Here's the drawing with two shaded views (mm, measured from the low corner). I have some questions. Round coordinates to 2 decimals unless told otherwise and drop trailing zeros. Order: outer loops, then holes, each group sorted by start corner. A loop starts at its lowest first (then second) coordinate and runs counter-clockwise, first axis right, second up. Notation, with made-up numbers: (68.5, 39) -> (127.5, 39) arc R27 cw to (127.5, 69) -> close; hole circle Ø7 at (-7, 69). An arc over 180 degrees is marked (long way). Use a Markdown table: item, result. Add a question column.
Q1. If we section it at A-A on y = 83: List the corners of the cut face in (x, z) for me (3 decimals), plus the area to 3 significant figures.
Q2. I'm going to push a flat-ended pin straight in: pin 1 Ø4 at (x, y) = (17, 192) entering from -Z. Where does the tip first touch, or does it pass through?
Q3. I need wall thicknesses on line 1 along Z through (x, y) = (15, 193.5) (3 decimals); line 2 along X through (y, z) = (268, 28.5). Which ranges of each line are inside material? Lowest first, please. Write a range as [from, to].
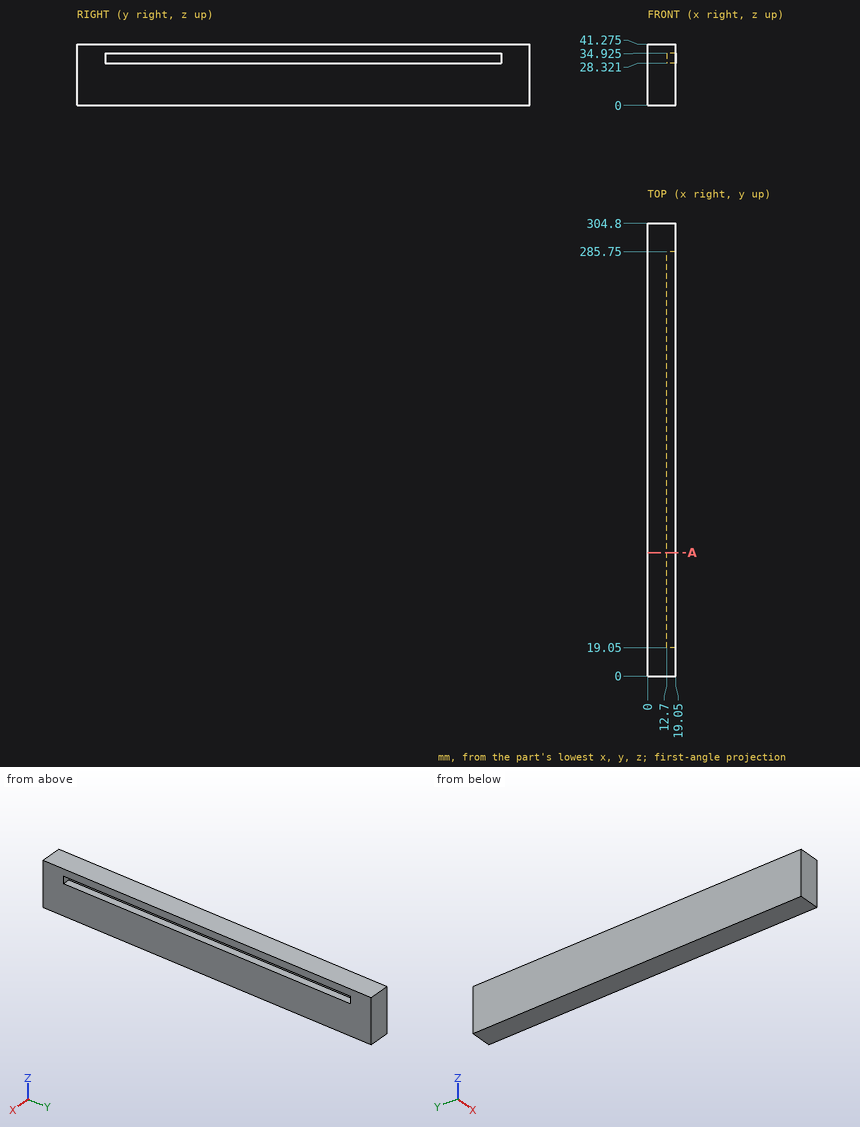
Answer below:
| question | item | result |
|---|---|---|
| 1 | outline | (0, 0) -> (19.05, 0) -> (19.05, 28.321) -> (12.7, 28.321) -> (12.7, 34.925) -> (19.05, 34.925) -> (19.05, 41.275) -> (0, 41.275) -> close |
| 1 | area | 744 mm² |
| 2 | pin 1 | z = 0 |
| 3 | line 1 | [0, 28.321], [34.925, 41.275] |
| 3 | line 2 | [0, 12.7] |
